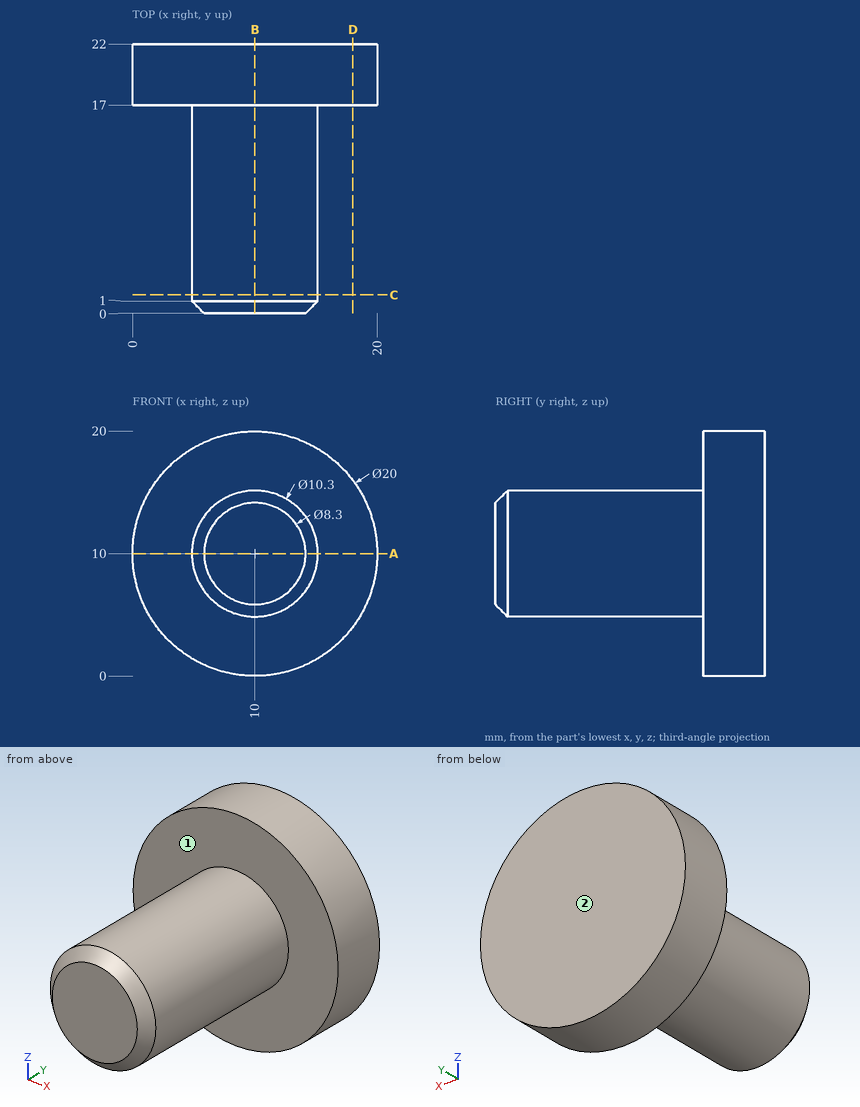
Job drawing, mm, ordinate dimensions from the low corner. One solid piece. A direction names the side the tool comes from. Coordinates: 2 decimals unless noted, no trailing zeros. Order: outer loops, then holes, each group sorted by start corner. A loop starts at its lowest first (then second) coordinate and runs counter-clockwise, first axis right, second up. Notation, with made-up numbers: (-13.75, -24) -> (-0.75, -24) arc R23 cw to (-0.75, 5) -> close; hole circle Ø2 at (43, -22.75). An arc over 180 degrees is marked (long way). Answer in a Markdown table with one row per item. Add a question column.
Q1. Band-saw the part on A-A, the plane z = 10. List the corners of the cut face in (x, y).
Q2. Band-saw the part on B-B, the plane x = 10. List the corners of the cut face in (y, z), then the cut area to 3 significant figures.
Q3. Which spindle directions (+Z, -Z, +X, -X, +Y, -Y) get a long thin tool onto all of the face, cutting with end or side? Do the marked faces 1 and 2. Say none if no direction does.
Q4. Wall check: line 1 along Y through (x, z) = (15.25, 9); line 2 along Z through (x, y) = (10.25, 10.75); line 3 along X through (y, z) = (16.5, 5.25). Give the ranges that are in metal, low to high. Write a range as [from, to].
Q5. Band-saw the part on D-D, the plane x = 18. List the corners of the cut face in (y, z).
Q6. Drop flat-ended pins along their axis: pin 1 (2 mm diameter, centred on x = 3, z = 13.5, fed in from -Y); pin 2 (8 mm diameter, centred on y = 16.5, z = 16.5, fed in from -X); pin 3 (2 mm diameter, centred on y = 12.5, z = 13, fed in from -X). Give the stop position or say it passes through.
Q7. Band-saw the part on C-C, the plane y = 1.5. List the corners of the cut face in (x, z).
Answers follow:
| question | item | result |
|---|---|---|
| 1 | outline | (0, 17) -> (4.85, 17) -> (4.85, 1) -> (5.85, 0) -> (14.15, 0) -> (15.15, 1) -> (15.15, 17) -> (20, 17) -> (20, 22) -> (0, 22) -> close |
| 2 | outline | (0, 5.85) -> (1, 4.85) -> (17, 4.85) -> (17, 0) -> (22, 0) -> (22, 20) -> (17, 20) -> (17, 15.15) -> (1, 15.15) -> (0, 14.15) -> close |
| 2 | area | 274 mm^2 |
| 3 | face 1 | -Y |
| 3 | face 2 | +Z, -Z, +X, -X, +Y |
| 4 | line 1 | [17, 22] |
| 4 | line 2 | [4.86, 15.14] |
| 4 | line 3 | [8.01, 11.99] |
| 5 | outline | (17, 4) -> (22, 4) -> (22, 16) -> (17, 16) -> close |
| 6 | pin 1 | y = 17 |
| 6 | pin 2 | x = 0.33 |
| 6 | pin 3 | x = 5.25 |
| 7 | outline | circle Ø10.3 at (10, 10) |
